```python
from build123d import *

# Parameters (mm, degrees)
SKETCH_1_W          = 12.5
SKETCH_1_H          = 22.4
EXTRUDE_1_DEPTH     = 30.9
SKETCH_4_W          = 31.8
SKETCH_4_H          = 2
EXTRUDE_2_DEPTH     = 12.5
SKETCH_6_R          = 1.5
CUT_EXTRUDE_2_DEPTH = 25.889405377
SKETCH_7_R          = 1.5
CUT_EXTRUDE_3_DEPTH = 3


with BuildPart() as part:
    # 草图1 → 凸台-拉伸1 (new body)
    with BuildSketch(Plane(origin=(0, 0, 0), x_dir=(1, 0, 0), z_dir=(0, 1, 0))):
        Rectangle(SKETCH_1_W, SKETCH_1_H)
    extrude(amount=EXTRUDE_1_DEPTH)

    # 草图4 → 凸台-拉伸2 (add)
    with BuildSketch(Plane(origin=(6.25, 0, 0), x_dir=(0, 0, -1), z_dir=(1, 0, 0))):
        with Locations((0, 17.1)):
            Rectangle(SKETCH_4_W, SKETCH_4_H)
    extrude(amount=-EXTRUDE_2_DEPTH)

    # 草图6 → 切除-拉伸2 (cut, through all)
    with BuildSketch(Plane(origin=(0, 18.1, 0), x_dir=(1, 0, 0), z_dir=(0, 1, 0))):
        with Locations(Location((0, 13.85, 0), (0, 0, 270))):
            Circle(SKETCH_6_R)
        with Locations(Location((0, -13.85, 0), (0, 0, 270))):
            Circle(SKETCH_6_R)
    extrude(amount=-CUT_EXTRUDE_2_DEPTH, mode=Mode.SUBTRACT)

    # 草图7 → 切除-拉伸3 (cut)
    with BuildSketch(Plane(origin=(0, 30.9, 0), x_dir=(1, 0, 0), z_dir=(0, 1, 0))):
        with Locations(Location((0, 5.2, 0), (0, 0, 270))):
            Circle(SKETCH_7_R)
    extrude(amount=-CUT_EXTRUDE_3_DEPTH, mode=Mode.SUBTRACT)


solid = part.part
```
Work out the finished part from the listing and answer in its coordinate system (mm). A direction names the side the tool comes from. Give positions to 0.01 mm unless a question says otherwise; leave off trailing zeros. Write each loop counter-clockwise with the first axis right and the second up, starting at its lowest first coordinate (ties: lowest second). Pieces come first, ordered by that corner, then holes.
(1) The part is cut by section B-B on x = 0. Write down the section's boundary in (y, z).
Final values:
outline: (0, -11.2) - (16.1, -11.2) - (16.1, -12.35) - (18.1, -12.35) - (18.1, -11.2) - (30.9, -11.2) - (30.9, -6.7) - (27.9, -6.7) - (27.9, -3.7) - (30.9, -3.7) - (30.9, 11.2) - (18.1, 11.2) - (18.1, 12.35) - (16.1, 12.35) - (16.1, 11.2) - (0, 11.2) - close; (16.1, -15.9) - (18.1, -15.9) - (18.1, -15.35) - (16.1, -15.35) - close; (16.1, 15.35) - (18.1, 15.35) - (18.1, 15.9) - (16.1, 15.9) - close
(2) Straight lines are drawn through the part: line 1 (X direction, y = 29.7, z = -5.2); line 2 (Z direction, x = -5.5, y = 28); line 3 (X direction, y = 17, z = -13). For each, find the intervals that lie inside material, in ascending order.
Final values:
line 1: x = -6.25 to -1.5, 1.5 to 6.25
line 2: z = -11.2 to 11.2
line 3: x = -6.25 to -1.24, 1.24 to 6.25
(3) The mould has two halves that part along X. Classify faces 1 (the cylindrical face through (0.07, 17.11, 12.35)), 2 (the flat face through (-6.25, 16, 0)), 3 (the flat face through (0, 30.9, 0)), 4 (the flat face through (6.25, 16, 0)): pulls with the +X half, pulls with the -X half, needs draft (parallel to the pull), parting line crosses it, or undercut.
Final values:
face 1: undercut
face 2: pulls with the -X half
face 3: needs draft
face 4: pulls with the +X half
(4) The part is cut by section C-C on x = 3.5. Write down the section's boundary in (y, z).
Final values:
outline: (0, -11.2) - (16.1, -11.2) - (16.1, -15.9) - (18.1, -15.9) - (18.1, -11.2) - (30.9, -11.2) - (30.9, 11.2) - (18.1, 11.2) - (18.1, 15.9) - (16.1, 15.9) - (16.1, 11.2) - (0, 11.2) - close
(5) The part is cut by section D-D on z = -5.2. Write down the section's boundary in (x, y), plus the area to 3 significant figures.
Final values:
outline: (-6.25, 0) - (6.25, 0) - (6.25, 30.9) - (1.5, 30.9) - (1.5, 27.9) - (-1.5, 27.9) - (-1.5, 30.9) - (-6.25, 30.9) - close
area: 377 mm2
(6) Which of the six approach directions +Z, -Z, +X, -X, +Y, -Y give full straight-line access (tool end or side, diameter ignored) to faces 5 (the flat face through (0, 8, -11.2)), 6 (the flat face through (0, 27.9, -5)), 7 (the flat face through (1.5, 18.1, -13)), 8 (the flat face through (1.5, 16.1, 13.1)), 9 (the flat face through (1.5, 18.1, 13.1))?
Final values:
face 5: -Z, +X, -X, -Y
face 6: +Y
face 7: -Z, +X, -X, +Y
face 8: +Z, +X, -X, -Y
face 9: +Z, +X, -X, +Y
(7) Flat-ended cylindrical pins translate along their axes: pin 1 Ø1.4 at (x, z) = (2.5, -13.5) entering from +Y; pin 2 Ø6 at (x, y) = (0, 7) entering from +Z; pin 3 Ø1.4 at (x, z) = (-0.5, 13.5) entering from -Y; pin 4 Ø4 at (x, y) = (2, 23) entering from -Z. Find the tip coordinate at first contact, or state that the pin passes through.
Final values:
pin 1: stops at y = 18.1
pin 2: stops at z = 11.2
pin 3: passes through
pin 4: stops at z = -11.2
(8) The part is cut by section A-A on z = 13.85. Write down the section's boundary in (x, y).
Final values:
outline: (-6.25, 16.1) - (-1.5, 16.1) - (-1.5, 18.1) - (-6.25, 18.1) - close; (1.5, 16.1) - (6.25, 16.1) - (6.25, 18.1) - (1.5, 18.1) - close
